from build123d import *

# Parameters (mm, degrees)
SKETCH1_W           = 50.8
SKETCH1_H           = 6.35
BOSS_EXTRUDE1_DEPTH = 5
SKETCH2_R           = 2
CUT_EXTRUDE1_DEPTH  = 5
CUT_EXTRUDE2_DEPTH  = 5


with BuildPart() as part:
    # Sketch1 → Boss-Extrude1 (new body)
    with BuildSketch(Plane.XY):
        with Locations((25.4, 3.175)):
            Rectangle(SKETCH1_W, SKETCH1_H)
    extrude(amount=BOSS_EXTRUDE1_DEPTH)

    # Sketch2 → Cut-Extrude1 (cut)
    with BuildSketch(Plane(origin=(0, 0, 0), x_dir=(-1, 0, 0), z_dir=(0, 0, -1))):
        with Locations((-6, 3.175)):
            Circle(SKETCH2_R)
    extrude(amount=-CUT_EXTRUDE1_DEPTH, mode=Mode.SUBTRACT)

    # Sketch3 → Cut-Extrude2 (cut)
    with BuildSketch(Plane(origin=(0, 0, 0), x_dir=(-1, 0, 0), z_dir=(0, 0, -1))):
        Polygon((-50.8, 0), (-16.807033998, 6.35), (-50.8, 6.35), align=None)
    extrude(amount=-CUT_EXTRUDE2_DEPTH, mode=Mode.SUBTRACT)


solid = part.part
Can you work these out from the model? Positions are in its coordinate system, mm. Round coordinates to 2 decimals unless told otherwise and drop trailing zeros. Order: outer loops, then holes, each group sorted by start corner. A loop starts at its lowest first (then second) coordinate and runs counter-clockwise, first axis right, second up. Notation, with made-up numbers: (74, -28) - (94, -28) arc R19 ccw to (94, -24) - close; hole circle Ø8 at (-17.75, 53). An arc over 180 degrees is marked (long way). Answer in a Markdown table with one row per item.
(1) Suppose I cut it at B-B, the plane y = 2.25. Please give me the cut outline in (x, z), plus the area to 3 significant figures.
From the geometry:
| item | result |
|---|---|
| outline | (0, 0) - (4.23, 0) - (4.23, 5) - (0, 5) - close; (7.77, 0) - (38.76, 0) - (38.76, 5) - (7.77, 5) - close |
| area | 176 mm2 |
(2) For P1, Ø1.5, axis at x = 36.5, y = 4, coming from the +Z side, with a flat end and sliding along its axis, tell me the tip position at first contact or that it passes through.
From the geometry:
| item | result |
|---|---|
| P1 | passes through |
(3) Suppose I cut it at A-A, the plane x = 6. Please give me the cut outline in (y, z) (3 decimals), plus the area to 4 significant figures.
From the geometry:
| item | result |
|---|---|
| outline | (0, 0) - (1.175, 0) - (1.175, 5) - (0, 5) - close; (5.175, 0) - (6.35, 0) - (6.35, 5) - (5.175, 5) - close |
| area | 11.75 mm2 |
(4) Suppose I cut it at C-C, the plane z = 2.4. Please give me the cut outline in (x, y) (3 decimals).
From the geometry:
| item | result |
|---|---|
| outline | (0, 0) - (50.8, 0) - (16.807, 6.35) - (0, 6.35) - close; hole circle Ø4 at (6, 3.175) |
(5) If we mould it in two halves opening along X, with no side actions, what happens to faces 1 (the face through (6.26, 5.16, 2.46)), 2 (the face through (34.04, 3.13, 2.46)), 3 (the face through (0, 3, 2)), 4 (the face through (19, 3, 0))? For each: released by +X, released by -X, zero draft, split by the parting line, or undercut.
From the geometry:
| item | result |
|---|---|
| face 1 | undercut |
| face 2 | released by +X |
| face 3 | released by -X |
| face 4 | zero draft |
(6) Please list where these lines run through material, in increasing order: L1, parallel to Y at x = 6, z = 1.35 (3 decimals); L2, parallel to Y at x = 44, z = 2; L3, parallel to Y at x = 23, z = 1.2. Write a range as from..to.
From the geometry:
| item | result |
|---|---|
| L1 | y = 0..1.175, 5.175..6.35 |
| L2 | y = 0..1.27 |
| L3 | y = 0..5.19 |
(7) Suppose I cut it at D-D, the plane x = 22.5. Please give me the cut outline in (y, z).
From the geometry:
| item | result |
|---|---|
| outline | (0, 0) - (5.29, 0) - (5.29, 5) - (0, 5) - close |
